The drawing under review shows one solid part. Ordinate dimensions are in mm from its lowest x, y, z. A direction names the side the tool comes from. Round coordinates to 2 decimals unless told otherwise and drop trailing zeros. Loops run counter-clockwise (first coordinate to the right, second up) from the corner with the lowest first, then second, coordinate; pieces in that order, holes last. Notation, with made-up numbers: (24, -21.75) -> (45, -21.75) arc R20 ccw to (45, 14.25) -> close; hole circle Ø7 at (19, 17.5). An arc over 180 degrees is marked (long way). Answer as CSV lines item,"result". Start each with the question number.
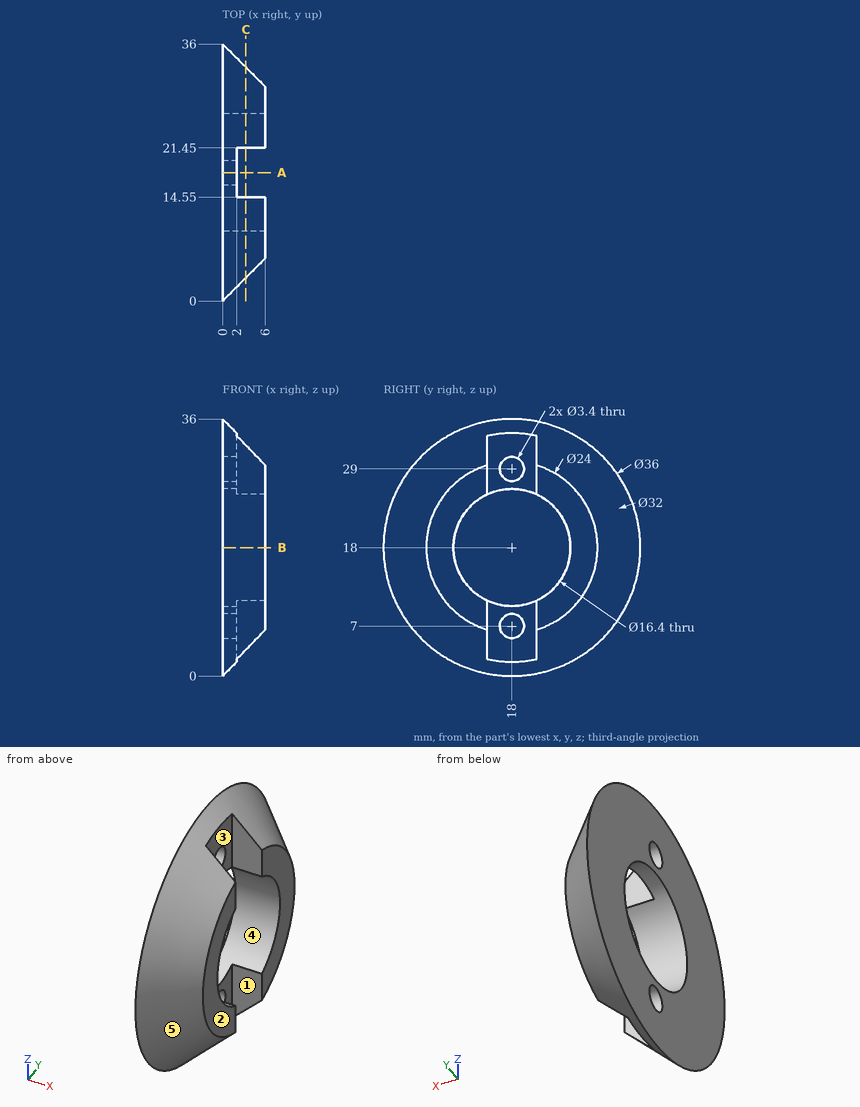
Q1. Machinability: for the marked faces 1 and 2, which of the approach directions +Z, -Z, +X, -X, +Y, -Y give a long, thin tool a straight path to every point of the face, cutting with its end or side? Answer none if there is none.
Q2. To check wall thickness, follow probe 1 along Z at (x, y) = (1.15, 18); probe 2 along Z at (x, y) = (5, 14.5); probe 3 along Z at (x, y) = (1, 14). State the ranges of each line that lie inside material, in increasing order. Write a range as from..to.
Q3. Add section C-C, the plane x = 3.25. Give the boundary of the cut face in (y, z), and give its area (3 significant figures).
Q4. Add section A-A, the plane y = 18. Give the boundary of the cut face in (x, z), and give its area (3 significant figures).
Q5. For pin 1 Ø2 at (x, y) = (2, 16.5) entering from +Z; pin 2 Ø3 at (x, z) = (4.5, 28.5) entering from +Y; pin 3 Ø2 at (x, z) = (4.5, 6) entering from -Y; pin 4 Ø2.5 at (y, z) = (18, 29) entering from +X (3 decimals), all flat-tipped, find the tip position at first contact; note any pin that passes through.
Q6. Add section B-B, the plane z = 18. Give the boundary of the cut face in (x, y), and give its area (3 significant figures).
Q7. Mouldability with a two-part tool opening along Z and no side actions: class the marked faces 3, 4 and 5 as pulls with the +Z half, pulls with the -Z half, needs draft (parallel to the pull), parting line crosses it, or undercut.
Worked answers:
1,face 1,"+Z, -Z, +X"
1,face 2,"+Z, -Z, +X, +Y, -Y"
2,probe 1,"z = 1.15..5.3, 8.7..9.8, 26.2..27.3, 30.7..34.85"
2,probe 2,"z = 5.48..10.58, 25.42..30.52"
2,probe 3,"z = 1.48..10.84, 25.16..34.52"
3,outline,"(14.55, 3.66) -> (14.55, 10.56) arc R8.2 cw to (14.55, 25.44) -> (14.55, 32.34) arc R14.75 ccw to start; (21.45, 3.66) arc R14.75 ccw to (21.45, 32.34) -> (21.45, 25.44) arc R8.2 cw to (21.45, 10.56) -> close"
3,area,"380 mm^2"
4,outline,"(0, 0) -> (2, 2) -> (2, 5.3) -> (0, 5.3) -> close; (0, 8.7) -> (2, 8.7) -> (2, 9.8) -> (0, 9.8) -> close; (0, 26.2) -> (2, 26.2) -> (2, 27.3) -> (0, 27.3) -> close; (0, 30.7) -> (2, 30.7) -> (2, 34) -> (0, 36) -> close"
4,area,"21.6 mm^2"
5,pin 1,"stops at z = 34.94"
5,pin 2,"stops at y = 29.14"
5,pin 3,"stops at y = 9.37"
5,pin 4,"passes through"
6,outline,"(0, 0) -> (6, 6) -> (6, 9.8) -> (0, 9.8) -> close; (0, 26.2) -> (6, 26.2) -> (6, 30) -> (0, 36) -> close"
6,area,"81.6 mm^2"
7,face 3,"needs draft"
7,face 4,"undercut"
7,face 5,"parting line crosses it"
